Can you work these out from the model? Positions are in its coordinate system, mm. A direction names the side the tool comes from. Give positions to 0.01 mm unless a question says otherwise; leave off trailing zeros. Write each loop counter-clockwise with the first axis right and the second up, starting at its lowest first coordinate (ties: lowest second). Pieces come first, ordered by that corner, then holes.
from build123d import *

# Parameters (mm, degrees)
SKETCH2_R           = 3.2639
BOSS_EXTRUDE1_DEPTH = 3.175


with BuildPart() as part:
    # Sketch2 → Boss-Extrude1 (new body)
    with BuildSketch(Plane(origin=(-112.555, 0, -573.58969557), x_dir=(0, 0.6231241879767124, 0.7821229100073485), z_dir=(-1, 0, 0))):
        with BuildLine():
            ThreePointArc((845.36792337, 140.568969032), (844.830619791, 138.700663745), (845.771780124, 136.999641403))
            Line((845.771780124, 136.999641403), (864.330586832, 122.213677187))
            ThreePointArc((864.330586832, 122.213677187), (874.263547789, 127), (884.196508746, 122.213677187))
            Line((884.196508746, 122.213677187), (887.735832346, 125.033487368))
            ThreePointArc((887.735832346, 125.033487368), (888.597587529, 126.330104481), (888.540958266, 127.885942216))
            Line((888.540958266, 127.885942216), (873.423706379, 169.576043207))
            ThreePointArc((873.423706379, 169.576043207), (871.446613669, 171.216745754), (869.04925283, 170.292915988))
            Line((869.04925283, 170.292915988), (863.47898249, 163.301314423))
            ThreePointArc((863.47898249, 163.301314423), (862.959009478, 162.129347633), (863.077713324, 160.852716328))
            Line((863.077713324, 160.852716328), (871.323924882, 138.111453883))
            ThreePointArc((871.323924882, 138.111453883), (871.188959814, 136.430204891), (869.830832527, 135.430052896))
            ThreePointArc((869.830832527, 135.430052896), (869.749583246, 135.412845003), (869.668400761, 135.39532469))
            ThreePointArc((869.668400761, 135.39532469), (868.550892206, 135.403510223), (867.545059791, 135.890535404))
            Line((867.545059791, 135.890535404), (853.685457311, 146.932602361))
            ThreePointArc((853.685457311, 146.932602361), (851.817152024, 147.46990594), (850.116129682, 146.528745607))
            Line((850.116129682, 146.528745607), (845.36792337, 140.568969032))
        make_face()
        with Locations((852.708507005, 139.592018726)):
            Circle(SKETCH2_R, mode=Mode.SUBTRACT)
        with Locations((869.774365973, 161.012466745)):
            Circle(SKETCH2_R, mode=Mode.SUBTRACT)
    extrude(amount=BOSS_EXTRUDE1_DEPTH)


solid = part.part
(1) Imagine slicing it at D-D, the plane z = 13.5. Write out the boundary of the cut face in (x, y) (3 decimals), plus the area to 3 significant figures.
Returned:
outline: (-115.73, 634.171) - (-112.555, 634.171) - (-112.555, 646.871) - (-115.73, 646.871) - close; (-115.73, 656.074) - (-112.555, 656.074) - (-112.555, 670.973) - (-115.73, 670.973) - close
area: 87.6 mm2
(2) Will these pins go through, and if not, where does the flat tip stop? P1, Ø1.5, axis at x = -114, z = 29, coming from the +Y side; P2, Ø5, axis at y = 640.52, z = 6.35, coming from the +X side.
Returned:
P1: stops at y = 661.93
P2: passes through
(3) Imagine slicing it at A-A, the plane y = 641. Write out the boundary of the cut face in (x, z) (3 decimals).
Returned:
outline: (-115.73, 0) - (-112.555, 0) - (-112.555, 3.121) - (-115.73, 3.121) - close; (-115.73, 9.579) - (-112.555, 9.579) - (-112.555, 28.261) - (-115.73, 28.261) - close
(4) Imagine slicing it at B-B, the plane z = 6.35. Write out the boundary of the cut face in (x, y) (3 decimals), plus the area to 3 significant figures.
Returned:
outline: (-115.73, 634.171) - (-112.555, 634.171) - (-112.555, 637.258) - (-115.73, 637.258) - close; (-115.73, 643.785) - (-112.555, 643.785) - (-112.555, 646.871) - (-115.73, 646.871) - close; (-115.73, 660.46) - (-112.555, 660.46) - (-112.555, 664.645) - (-115.73, 664.645) - close; (-115.73, 671.173) - (-112.555, 671.173) - (-112.555, 675.358) - (-115.73, 675.358) - close
area: 46.2 mm2
(5) Imagine slicing it at C-C, the plane x = -114. Write out the boundary of the cut face in (y, z), plus the area to 3 significant figures.
Returned:
outline: (634.17, 2.54) arc R2.54 ccw to (636.71, 0) - (644.33, 0) arc R2.54 ccw to (646.87, 2.54) - (646.87, 20.26) arc R2.54 cw to (647.81, 22.23) arc R21.59 ccw to (647.94, 22.34) arc R2.03 cw to (650.96, 21.83) - (663.61, 1.21) arc R2.54 ccw to (665.78, 0) - (674.72, 0) arc R2.54 ccw to (676.88, 3.87) - (653.69, 41.67) arc R2.54 ccw to (650.96, 42.82) - (646.55, 41.81) arc R12.7 cw to (634.17, 26.27) - close; hole circle Ø6.53 at (640.52, 6.35); hole circle Ø6.53 at (667.91, 6.35)
area: 878 mm2
(6) For faces 4 (the face through (-114.12, 676.95, 1.33)), 5 (the face through (-114.12, 647.12, 21.36)), which set-ups out of +Z, -Z, +X, -X, +Y, -Y let a thin tool reach every point of the face, with its end or its side?
Returned:
face 4: +X, -X, +Y
face 5: -Z, +X, -X
(7) If we mould it in two halves opening along Y, with no side actions, what happens to faces 1 (the face through (-114.1, 648.7, 42.3)), 2 (the face through (-114.12, 657.376, 11.378)), 3 (the face through (-114, 641, 0))? For each: +Y half, -Y half, draft (parallel to the pull), parting line (faces both ways), or undercut.
Returned:
face 1: -Y half
face 2: undercut
face 3: draft
(8) If I drill on L1, parallel to Y at x = -114.55, z = 6.35; L2, parallel to Y at x = -113.85, z = 5.5; L3, parallel to Y at x = -114.5, z = 18, over which ranges is the centre line in solid material (lowest first)?
Returned:
L1: y = 634.17 to 637.26, 643.79 to 646.87, 660.46 to 664.65, 671.17 to 675.36
L2: y = 634.17 to 637.37, 643.67 to 646.87, 660.98 to 664.76, 671.06 to 675.88
L3: y = 634.17 to 646.87, 653.31 to 668.21
